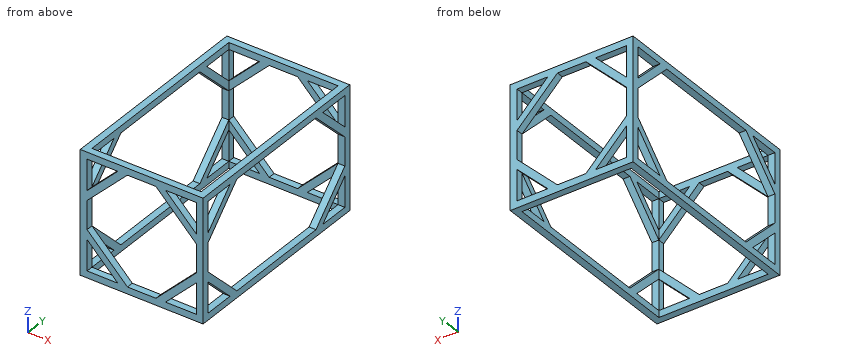
```python
from build123d import *

# Parameters (mm, degrees)
F0_W     = 914.4
F0_H     = 1524
F1_DEPTH = 914.4
F3_DEPTH = 2540
F5_DEPTH = 2540
F7_DEPTH = 914.4


with BuildPart() as f1:
    # F0 (on Top) → F1 (new body)
    with BuildSketch(Plane.XY):
        with Locations((457.2, 762)):
            Rectangle(F0_W, F0_H)
    extrude(amount=F1_DEPTH)

    # F2 (on Right) → F3 (cut)
    with BuildSketch(Plane.YZ):
        Polygon((1244.6, 863.6), (1473.2, 635), (1473.2, 863.6), align=None)
        Polygon((1244.6, 50.8), (1473.2, 50.8), (1473.2, 279.4), align=None)
        Polygon((1172.757951, 50.8), (1473.2, 351.242049), (1473.2, 563.157951), (1172.757951, 863.6), (351.242049, 863.6), (50.8, 563.157951), (50.8, 351.242049), (351.242049, 50.8), align=None)
        Polygon((50.8, 635), (279.4, 863.6), (50.8, 863.6), align=None)
        Polygon((50.8, 50.8), (279.4, 50.8), (50.8, 279.4), align=None)
    extrude(amount=F3_DEPTH, mode=Mode.SUBTRACT)

    # F4 (on Front) → F5 (cut)
    with BuildSketch(Plane.XZ):
        Polygon((50.8, 351.242049), (351.242049, 50.8), (563.157951, 50.8), (863.6, 351.242049), (863.6, 563.157951), (563.157951, 863.6), (351.242049, 863.6), (50.8, 563.157951), align=None)
        Polygon((50.8, 863.6), (50.8, 635), (279.4, 863.6), align=None)
        Polygon((50.8, 279.4), (50.8, 50.8), (279.4, 50.8), align=None)
        Polygon((863.6, 279.4), (635, 50.8), (863.6, 50.8), align=None)
        Polygon((635, 863.6), (863.6, 635), (863.6, 863.6), align=None)
    extrude(amount=-F5_DEPTH, mode=Mode.SUBTRACT)

    # F6 (on face) → F7 (cut)
    with BuildSketch(Plane.XY.offset(914.4)):
        Polygon((50.8, 1473.2), (50.8, 1472.929239), (50.8, 50.8), (863.6, 50.8), (863.6, 1473.2), align=None)
    extrude(amount=-F7_DEPTH, mode=Mode.SUBTRACT)


solid = f1.part
```
For this review, take the finished solid that the model builds, in its own axes (mm). Coordinates: 2 decimals unless noted, no trailing zeros. Loops run counter-clockwise (first coordinate to the right, second up) from the corner with the lowest first, then second, coordinate; pieces in that order, holes last. Notation, with made-up numbers: (66.25, 79) -> (72.25, 79) arc R12 ccw to (72.25, 98) -> close; hole circle Ø8 at (86.25, 54). An arc over 180 degrees is marked (long way). Return JSON: item names as keys, results as strings. Group by question number.
(1) Consider section A-A, the plane z = 480. Give the boundary of the cut face in (x, y), plus the area to 3 significant figures.
(2) To check wall thickness, follow L1, parallel to X at y = 117, z = 662.5; L2, parallel to Y at x = 452, z = 867. State the ranges of each line that lie inside material, in increasing order.
(3) Consider section B-B, the plane y = 867. Give the boundary of the cut face in (x, z).
(4) Consider section C-C, the plane x = 239. Count the separate pieces of the cut face and the enclosed holes in it, plus the area to 3 significant figures.
Results below:
{
 "1": {"outline": "(0, 0) -> (50.8, 0) -> (50.8, 50.8) -> (0, 50.8) -> close; (0, 1473.2) -> (50.8, 1473.2) -> (50.8, 1524) -> (0, 1524) -> close; (863.6, 0) -> (914.4, 0) -> (914.4, 50.8) -> (863.6, 50.8) -> close; (863.6, 1473.2) -> (914.4, 1473.2) -> (914.4, 1524) -> (863.6, 1524) -> close", "area": "10,300 mm2"},
 "2": {"L1": "x = 0 to 50.8, 863.6 to 914.4", "L2": "y = 0 to 50.8, 1473.2 to 1524"},
 "3": {"outline": "(0, 0) -> (50.8, 0) -> (50.8, 50.8) -> (0, 50.8) -> close; (0, 863.6) -> (50.8, 863.6) -> (50.8, 914.4) -> (0, 914.4) -> close; (863.6, 0) -> (914.4, 0) -> (914.4, 50.8) -> (863.6, 50.8) -> close; (863.6, 863.6) -> (914.4, 863.6) -> (914.4, 914.4) -> (863.6, 914.4) -> close"},
 "4": {"separate pieces": "8", "enclosed holes": "0", "area": "24,900 mm2"}
}
